The listing builds one solid part. Answer for the finished solid, in the listing's coordinates (mm). Face numbers are marked on the shaded views. A direction names the side the tool comes from. Give positions to 0.01 mm unless a question says otherwise; leave off trailing zeros. Loops run counter-clockwise (first coordinate to the right, second up) from the corner with the lowest first, then second, coordinate; pieces in that order, holes last. Notation, with made-up numbers: (51.25, 79.25) - (55.25, 79.25) arc R24 ccw to (55.25, 104.25) - close; hole circle Ø1 at (19.5, 55.25). An arc over 180 degrees is marked (long way). Write each question's results on one line, items separated by ' | '.
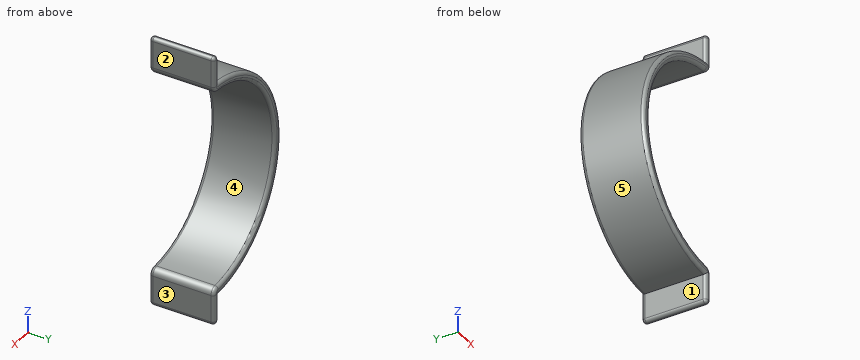
Autodesk Inventor part; units mm, degrees
ref_plane "YZ Plane" through (0, 0, 0) normal (1, 0, 0) x (0, 1, 0)
ref_plane "XZ Plane" through (0, 0, 0) normal (0, 1, 0) x (-1, 0, 0)
ref_plane "XY Plane" through (0, 0, 0) normal (0, 0, 1) x (1, 0, 0)
sketch "Sketch1" plane through (0, 0, 0) normal (0, 1, 0) x (-1, 0, 0)
  line L0 (0, 0) -> (0, -100)
  line L1 (0, -50) -> (50, -50)
  circle A0 centre (0, -50) radius 50
  line L2 (50, -50) -> (46, -50)
  line L3 (0, 0) -> (0, 13)
  line L4 (0, -100) -> (0, -113)
  circle A1 centre (0, -50) radius 46
  line L5 (0, 13) -> (3, 13)
  line L6 (3, 13) -> (3, -0.99065)
  line L7 (3, -0.99065) -> (0, -0.99065)
  line L8 (0, -0.99065) -> (0, 13)
  line L9 (0, -113) -> (3, -113)
  line L10 (3, -113) -> (3, -98.99687)
  line L11 (3, -98.99687) -> (0, -98.99687)
  line L12 (0, -98.99687) -> (0, -113)
  point P0 (0, -4)
  point P1 (0, -96)
  point P2 (3, -99.909919)
  point P3 (3, -0.090081)
  dimension "d0" = 100
  dimension "d1" = 50
  dimension "d2" = 4
  dimension "d3" = 13
  dimension "d4" = 13
  dimension "d5" = 3
  dimension "d6" = 3
sketch "Sketch1 outline for Extrusion1" plane through (0, 0, 0) normal (0, 1, 0) x (-1, 0, 0)
  line L0 (3, 13) -> (0, 13)
  line L1 (3, -0.090081) -> (3, 13)
  arc A0 (3, -99.909919) -> (3, -0.090081) centre (0, -50) ccw
  line L2 (3, -113) -> (3, -99.909919)
  line L3 (0, -113) -> (3, -113)
  line L4 (0, -100) -> (0, -113)
  line L5 (0, -96) -> (0, -100)
  arc A1 (0, -4) -> (0, -96) centre (0, -50) cw
  line L6 (0, 0) -> (0, -4)
  line L7 (0, 13) -> (0, 0)
extrude "Extrusion1" add sketch "Sketch1 outline for Extrusion1" along normal blind 30
fillet "Fillet1" radius 3.175 2 edges at (0, 15, -96) (0, 15, -4)
fillet "Fillet2" radius 1.5 4 edges at (-3, 15, 13) (0, 15, 13) (-3, 15, -113) (0, 15, -113)
fillet "Fillet3" radius 1.5 20 edges at (-0.8586, 30, -96.901) (-0.8586, 30, -3.099) (0, 30, -99.5362) (0, 30, -0.4638) (-2.5607, 30, -112.5607) (-3, 30, -105.705) (-2.5607, 30, 12.5607) (-3, 30, 5.705) (-46, 30, -50) (-50, 30, -50) (-0.8586, 0, -96.901) (-0.8586, 0, -3.099) (0, 0, -99.5362) (0, 0, -0.4638) (-2.5607, 0, -112.5607) (-3, 0, -105.705) (-2.5607, 0, 12.5607) (-3, 0, 5.705) (-46, 0, -50) (-50, 0, -50)
properties part number "handle"
Item 1: A cutting plane is placed at A-A, the plane z = -50. Determine the outline of the cut face in (x, y).
Values found:
outline: (-50, 1.5) arc R1.5 ccw to (-48.5, 0) - (-47.5, 0) arc R1.5 ccw to (-46, 1.5) - (-46, 28.5) arc R1.5 ccw to (-47.5, 30) - (-48.5, 30) arc R1.5 ccw to (-50, 28.5) - close
Item 2: Find the intervals of material crossed by line 1 along X through (y, z) = (21.5, -49.5); line 2 along Z through (x, y) = (-33, 23); line 3 along Z through (x, y) = (-9.5, 15.5), in increasing order. Write a range as [from, to].
Values found:
line 1: x = [-50, -46] | line 2: z = [-87.56, -82.05], [-17.95, -12.44] | line 3: z = [-99.09, -95.01], [-4.99, -0.91]
Item 3: For a pull along Z with two mould halves and no side action, classify the marked faces 3, 4 and 5 as released by +Z, released by -Z, zero draft, split by the parting line, or undercut.
Values found:
face 3: zero draft | face 4: undercut | face 5: split by the parting line
Item 4: Flat-ended cylindrical pins translate along their axes: P1, Ø6, axis at x = -18, y = 14.5, coming from the -Z side; P2, Ø1, axis at x = -16.5, y = 26, coming from the +Z side; P3, Ø12, axis at y = 12.5, z = -58.5, coming from the -X side. Find the tip coordinate at first contact, or state that the pin passes through.
Values found:
P1: stops at z = -97.7 | P2: stops at z = -2.63 | P3: stops at x = -49.94
Item 5: For the marked faces 1 and 2, determine the directions among +Z, -Z, +X, -X, +Y, -Y from which every point of the face is accessible in a straight line to the end or side of a thin tool.
Values found:
face 1: -Z, -X, +Y, -Y | face 2: +Z, -Z, +X, +Y, -Y
